Study the drawing (mm; zero at the part's minimum x, y, z) and answer. A direction names the side the tool comes from. Coordinates: 2 decimals unless noted, no trailing zeros. Loops run counter-clockwise (first coordinate to the right, second up) from the corner with the lowest first, then second, coordinate; pieces in that order, holes last. Notation, with made-up numbers: (38, 76) -> (83, 76) arc R17 ccw to (83, 87) -> close; hole circle Ø11 at (4, -37.5). An arc over 180 degrees is marked (long way). Answer as a JSON object with one key per item and string values. Group by question number.
Q1. Determine the mould class of the marked faces 1, 2 and 3 for opening direction X: released by +X, released by -X, zero draft, split by the parting line, or undercut.
Q2. Each of these flat-tipped pins is pushed along its axis until it touches: P1, Ø1.5, axis at y = 11, z = 8.5, coming from the -X side; P2, Ø5.5, axis at x = 8.5, z = 8.5, coming from the -Y side. Where does it stop, or does it pass through?
Q3. The part is cut by section A-A on x = 7.5. Write down the section's boundary in (y, z) (1 decimal), and give its area (3 significant figures).
Q4. Straight lines are drawn through the part: line 1 along X through (y, z) = (2.1, 7); line 2 along Y through (x, z) = (7.5, 5) (1 decimal); line 3 along X through (y, z) = (7, 10) (1 decimal). For each, find the intervals that lie inside material, in ascending order. Write a range as [from, to].
Q5. For the marked faces 4 and 5, determine the directions among +Z, -Z, +X, -X, +Y, -Y from which every point of the face is accessible in a straight line to the end or side of a thin tool.
Q6. The part is cut by section D-D on y = 6.75. Write down the section's boundary in (x, z), and give its area (3 significant figures).
Q7. The part is cut by section C-C on y = 2.25. Write down the section's boundary in (x, z), and give its area (3 significant figures).
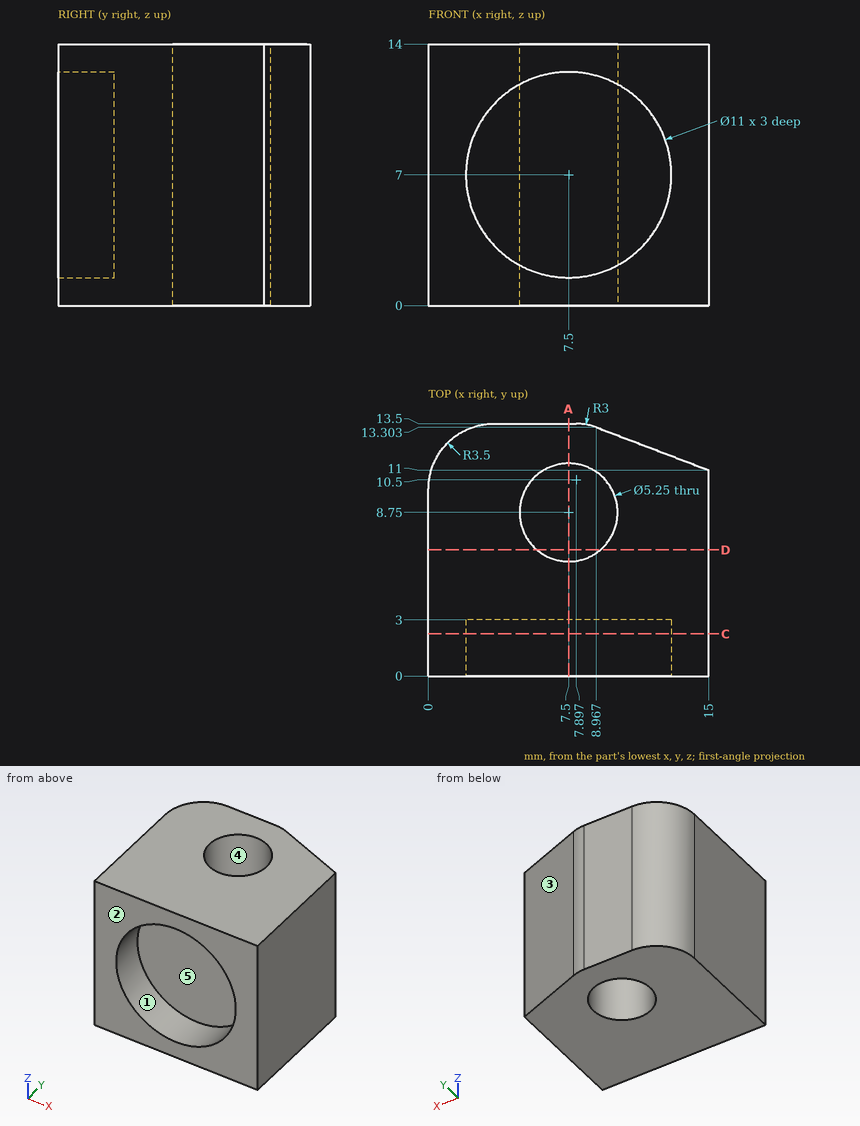
Final values:
{
 "1": {"face 1": "undercut", "face 2": "zero draft", "face 3": "released by +X"},
 "2": {"P1": "stops at x = 0.01", "P2": "stops at y = 3"},
 "3": {"outline": "(0, 0) -> (6.1, 0) -> (6.1, 14) -> (0, 14) -> (0, 12.5) -> (3, 12.5) -> (3, 1.5) -> (0, 1.5) -> close; (11.4, 0) -> (13.5, 0) -> (13.5, 14) -> (11.4, 14) -> close", "area": "82.5 mm2"},
 "4": {"line 1": "x = [0, 2], [13, 15]", "line 2": "y = [3, 6.1], [11.4, 13.5]", "line 3": "x = [0, 5.5], [9.5, 15]"},
 "5": {"face 4": "+Z, -Z", "face 5": "-Y"},
 "6": {"outline": "(0, 0) -> (5.8, 0) -> (5.8, 14) -> (0, 14) -> close; (9.2, 0) -> (15, 0) -> (15, 14) -> (9.2, 14) -> close", "area": "162 mm2"},
 "7": {"outline": "(0, 0) -> (15, 0) -> (15, 14) -> (0, 14) -> close; hole circle Ø11 at (7.5, 7)", "area": "115 mm2"}
}
